Source: CAD feature listing. Evaluate the final solid. Frame: model axes, mm. Face numbers are marked on the shaded views. A direction names the side the tool comes from. Round coordinates to 2 decimals unless told otherwise and drop trailing zeros. Loops run counter-clockwise (first coordinate to the right, second up) from the corner with the lowest first, then second, coordinate; pieces in that order, holes last. Notation, with made-up numbers: (58.5, -7.75) - (84.5, -7.75) arc R13 ccw to (84.5, -0.75) - close; hole circle Ø4 at (52, 19). An arc over 180 degrees is marked (long way). Use CSV: the item, a comma, the result in double quotes. Start each with the question number.
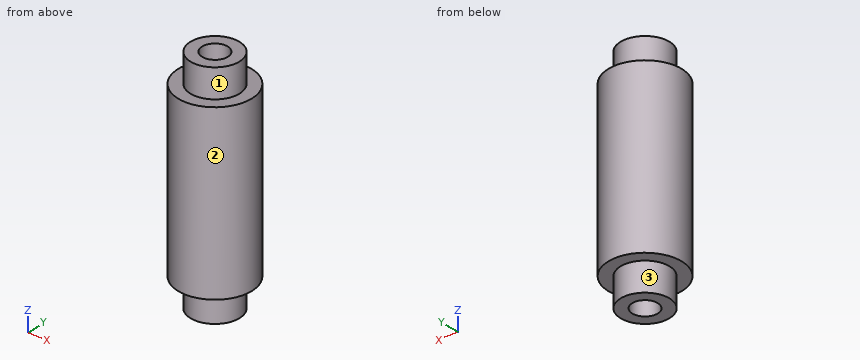
Autodesk Inventor part; units mm, degrees
ref_plane "Work Plane1" through (0, 0, 6.35) normal (0, 0, 1) x (1, 0, 0)
ref_plane "YZ Plane" through (0, 0, 0) normal (1, 0, 0) x (0, 1, 0)
ref_plane "XZ Plane" through (0, 0, 0) normal (0, 1, 0) x (-1, 0, 0)
sketch "Sketch1" plane through (0, 0, 0) normal (0, 0, 1) x (1, 0, 0)
  circle A0 centre (0, 0) radius 7.1437
  dimension "d0" = 14.2875
extrude "Extrusion1" add sketch "Sketch1" along normal blind 33.3375
ref_plane "Work Plane1" through (0, 0, 6.35) normal (0, 0, 1) x (1, 0, 0)
sketch "Sketch6" plane through (0, 0, 33.3375) normal (0, 0, 1) x (1, 0, 0)
  circle A0 centre (0, 0) radius 2.4892
  dimension "d28" = 4.9784
extrude "Extrusion3" cut sketch "Sketch6" against normal through all
sketch "Sketch7" plane through (0, 0, 33.3375) normal (0, 0, 1) x (1, 0, 0)
  circle A0 centre (0, 0) radius 4.7625
  circle A1 centre (0, 0) radius 2.4892
  dimension "d31" = 9.525
  dimension "d32" = 4.9784
extrude "Extrusion4" add sketch "Sketch7" along normal blind 5.5563
sketch "Sketch8" plane through (0, 0, 0) normal (0, 0, -1) x (-1, 0, 0)
  circle A0 centre (0, 0) radius 2.4892
  circle A1 centre (0, 0) radius 4.7625
extrude "Extrusion5" add sketch "Sketch8" along normal blind 5.5563
ref_plane "Work Plane2" through (0, 0, 16.6688) normal (0, 0, 1) x (1, 0, 0)
properties part number "RollerSpacer2(Bearing)"
1. Contact query for flat-ended pins moving along their axis: P1, Ø3, axis at y = 5, z = 17, coming from the -X side; P2, Ø8, axis at x = 0, y = 0, coming from the +Z side; P3, Ø1.5, axis at y = -3, z = 25.5, coming from the +X side; P4, Ø1.5, axis at y = -1.5, z = 18, coming from the +X side. Output: stop coordinate, or through.
2. Section query D-D on y = -3.75. Return the cut outline in (x, z), and give its area (3 significant figures).
3. Section query A-A on y = 0. Return the cut outline in (x, z).
4. Line query: line 1 along Y through (x, z) = (0, 17); line 2 along Y through (x, z) = (0, 34.5); line 3 along Z through (x, y) = (-2.5, 4.25). Output: solid intervals per line, ascending.
5. Reachability of the marked faces 1, 2 and 3 from +Z, -Z, +X, -X, +Y, -Y: full face, straight path, thin tool, end or side. Return the list, or none.
6. Section query C-C on z = 6.5. Return the cut outline in (x, y).
Values:
1,P1,"stops at x = -6.23"
1,P2,"stops at z = 38.89"
1,P3,"stops at x = 6.78"
1,P4,"stops at x = 7.1"
2,outline,"(-6.08, 0) - (-2.94, 0) - (-2.94, -5.56) - (2.94, -5.56) - (2.94, 0) - (6.08, 0) - (6.08, 33.34) - (2.94, 33.34) - (2.94, 38.89) - (-2.94, 38.89) - (-2.94, 33.34) - (-6.08, 33.34) - close"
2,area,"471 mm^2"
3,outline,"(-7.14, 0) - (-4.76, 0) - (-4.76, -5.56) - (-2.49, -5.56) - (-2.49, 38.89) - (-4.76, 38.89) - (-4.76, 33.34) - (-7.14, 33.34) - close; (2.49, -5.56) - (4.76, -5.56) - (4.76, 0) - (7.14, 0) - (7.14, 33.34) - (4.76, 33.34) - (4.76, 38.89) - (2.49, 38.89) - close"
4,line 1,"y = -7.14 to -2.49, 2.49 to 7.14"
4,line 2,"y = -4.76 to -2.49, 2.49 to 4.76"
4,line 3,"z = 0 to 33.34"
5,face 1,"+Z"
5,face 2,"+Z, -Z"
5,face 3,"-Z"
6,outline,"circle Ø14.29 at (0, 0); hole circle Ø4.98 at (0, 0)"
